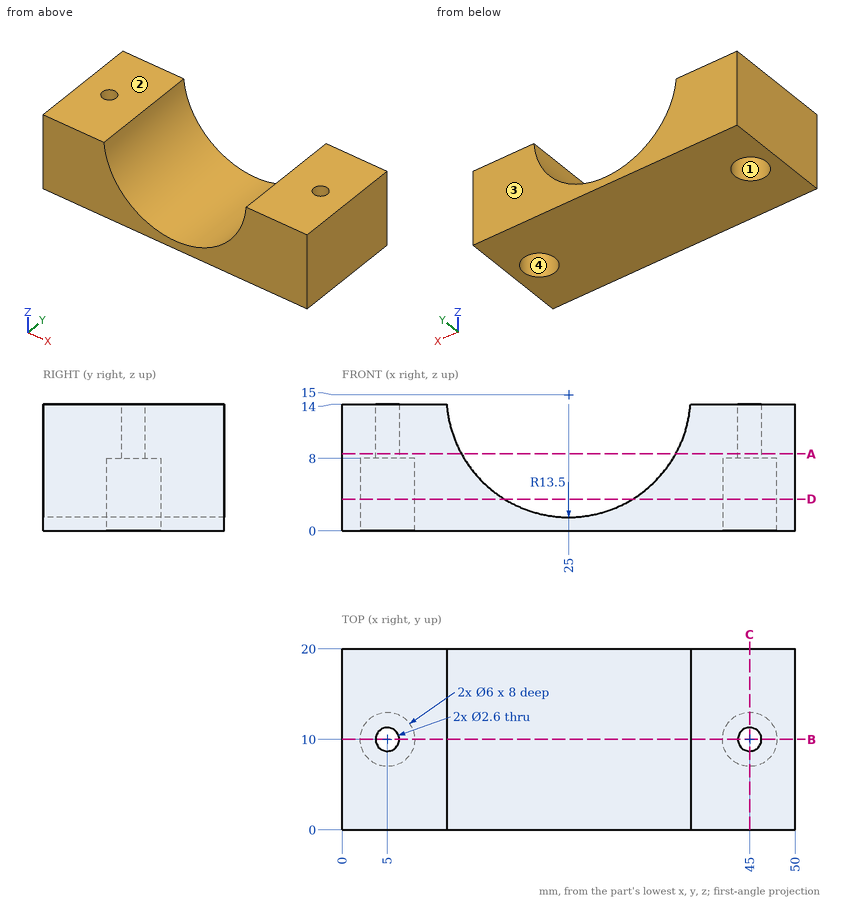
Verification items for this drawing (mm, ordinates from the low corner). Coordinates: 2 decimals unless noted, no trailing zeros. Order: outer loops, then holes, each group sorted by start corner. A loop starts at its lowest first (then second) coordinate and runs counter-clockwise, first axis right, second up. Notation, with made-up numbers: M -8,3.5 L 44,3.5 A32 cw 44,40.5 Z; hole C 70.25,-5.75 d9. An arc over 180 degrees is marked long. One line per item, written item: value. Start each with the question number.
Item 1: Sectioned sample at B-B on y = 10. Record the cut outline in (x, z), then the cut area to 3 significant figures.
Item 2: Sectioned sample at D-D on z = 3.5. Record the cut outline in (x, y).
Item 3: Mould release check, pull along Y, two halves, no side actions. Record for the marked faces 1, 2, 3 and 4: pulls with the +Y half, pulls with the -Y half, needs draft (parallel to the pull), parting line crosses it, or undercut.
Item 4: Depth check by flat-ended pin: P1, Ø2, axis at x = 38, y = 9.5, coming from the -Z side; P2, Ø3, axis at x = 4, y = 9, coming from the -Z side; P3, Ø4, axis at x = 17, y = 7, coming from the +Z side. Enter the tip coordinate at first touch or a pass-through.
Item 5: Sectioned sample at C-C on x = 45. Record the cut outline in (y, z).
Item 6: Sectioned sample at A-A on z = 8.5. Record the cut outline in (x, y).
Item 7: Thickness scan on probe 1 along Y at (x, z) = (45, 10.5); probe 2 along X at (y, z) = (7.5, 7.25); probe 3 along Y at (x, z) = (45, 6). Record the ranges inside material, lowest first.
Calculated:
1. outline: M 0,0 L 2,0 L 2,8 L 3.7,8 L 3.7,14 L 0,14 Z; M 6.3,8 L 8,8 L 8,0 L 42,0 L 42,8 L 43.7,8 L 43.7,14 L 38.46,14 A13.5 cw 11.54,14 L 6.3,14 Z; M 46.3,8 L 48,8 L 48,0 L 50,0 L 50,14 L 46.3,14 Z
1. area: 313 mm^2
2. outline: M 0,0 L 17.93,0 L 17.93,20 L 0,20 Z; M 32.07,0 L 50,0 L 50,20 L 32.07,20 Z; hole C 5,10 d6; hole C 45,10 d6
3. face 1: undercut
3. face 2: needs draft
3. face 3: pulls with the +Y half
3. face 4: undercut
4. P1: z = 0
4. P2: z = 8
4. P3: z = 5.93
5. outline: M 0,0 L 7,0 L 7,8 L 8.7,8 L 8.7,14 L 0,14 Z; M 11.3,8 L 13,8 L 13,0 L 20,0 L 20,14 L 11.3,14 Z
6. outline: M 0,0 L 13.17,0 L 13.17,20 L 0,20 Z; M 36.83,0 L 50,0 L 50,20 L 36.83,20 Z; hole C 5,10 d2.6; hole C 45,10 d2.6
7. probe 1: 0 to 8.7, 11.3 to 20
7. probe 2: 0 to 3.34, 6.66 to 13.95, 36.05 to 43.34, 46.66 to 50
7. probe 3: 0 to 7, 13 to 20
